Verification items for this drawing (mm, ordinates from the low corner). A direction names the side the tool comes from. Coordinates: 2 decimals unless noted, no trailing zeros. Write each loop counter-clockwise with the first axis right and the second up, starting at its lowest first coordinate (ties: lowest second). Pieces come first, ordered by that corner, then holes. Notation, with made-up numbers: M -14,66.5 L 38,66.5 A21 cw 38,81.5 Z; hole C 56,1 d7. An arc over 180 degrees is marked long. Write each question's results on one line, items separated by ' | '.
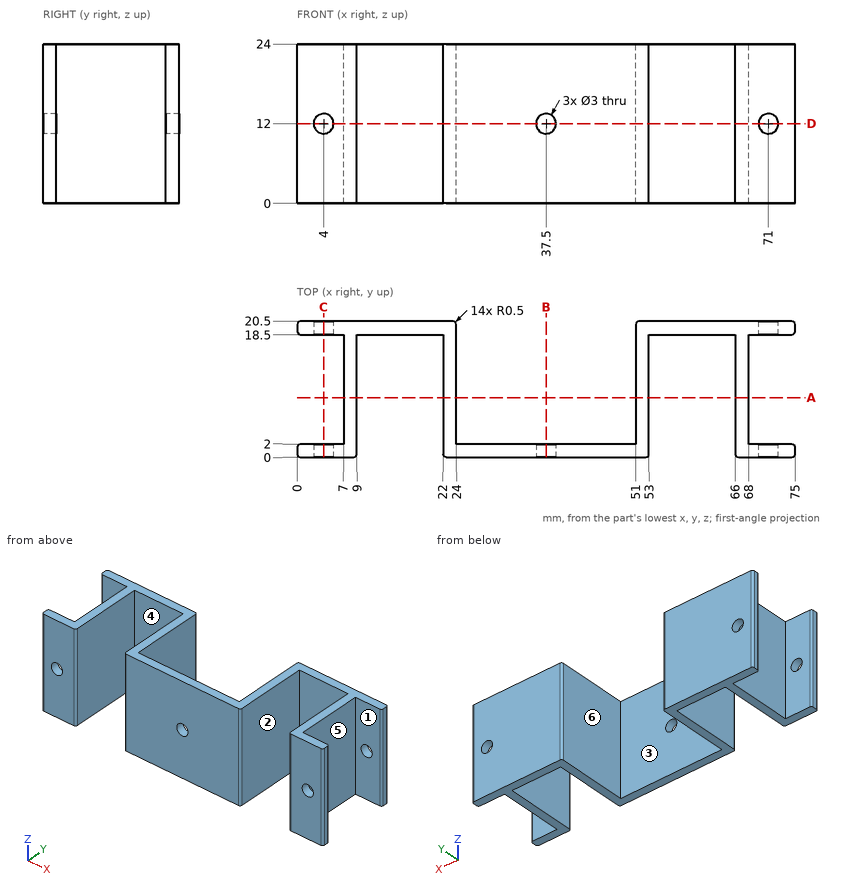
Q1. Scan lines: probe 1 along X at (y, z) = (8.5, 2); probe 2 along X at (y, z) = (1.5, 4.5); probe 3 along Z at (x, y) = (37.5, 0.85). Record each from-to range of solid material in increasing order.
Geometry check:
probe 1: x = 7 to 9, 22 to 24, 51 to 53, 66 to 68 | probe 2: x = 0 to 9, 22 to 53, 66 to 75 | probe 3: z = 0 to 10.5, 13.5 to 24
Q2. Sectioned sample at D-D on z = 12. Give the number of separate pieces and of enclosed holes in the cut face, and give its area (3 significant figures).
Geometry check:
separate pieces: 6 | enclosed holes: 0 | area: 295 mm2
Q3. Mould release check, pull along Y, two halves, no side actions. Record for the marked faces 4, 5 and 6: pulls with the +Y half, pulls with the -Y half, needs draft (parallel to the pull), parting line crosses it, or undercut.
Geometry check:
face 4: pulls with the -Y half | face 5: undercut | face 6: needs draft
Q4. Sectioned sample at A-A on y = 9. Record the cut outline in (x, z), and give its area (3 significant figures).
Geometry check:
outline: M 7,0 L 9,0 L 9,24 L 7,24 Z; M 22,0 L 24,0 L 24,24 L 22,24 Z; M 51,0 L 53,0 L 53,24 L 51,24 Z; M 66,0 L 68,0 L 68,24 L 66,24 Z | area: 192 mm2
Q5. Depth check by flat-ended pin: P1, Ø2, axis at y = 11.5, z = 15, coming from the -X side; P2, Ø8, axis at y = 8.5, z = 19.5, coming from the +X side; P3, Ø4, axis at x = 14.5, z = 7, coming from the -Y side; P4, Ø12, axis at x = 42, y = 13.5, coming from the -Z side. Enter the tip coordinate at first touch or a pass-through.
Geometry check:
P1: stops at x = 7 | P2: stops at x = 68 | P3: stops at y = 18.5 | P4: passes through
Q6. Sectioned sample at C-C on x = 4. Record the cut outline in (y, z), and give its area (3 significant figures).
Geometry check:
outline: M 0,0 L 2,0 L 2,10.5 L 0,10.5 Z; M 0,13.5 L 2,13.5 L 2,24 L 0,24 Z; M 18.5,0 L 20.5,0 L 20.5,10.5 L 18.5,10.5 Z; M 18.5,13.5 L 20.5,13.5 L 20.5,24 L 18.5,24 Z | area: 84.0 mm2
Q7. Sectioned sample at B-B on x = 37.5. Record the cut outline in (y, z), and give its area (3 significant figures).
Geometry check:
outline: M 0,0 L 2,0 L 2,10.5 L 0,10.5 Z; M 0,13.5 L 2,13.5 L 2,24 L 0,24 Z | area: 42.0 mm2
Q8. Access from +Z, -Z, +X, -X, +Y, -Y to the whole of each face (thin tool, end or side, straight path). Record for the marked faces 1, 2 and 3.
Geometry check:
face 1: +Z, -Z, +X | face 2: +Z, -Z, -Y | face 3: +Z, -Z, +Y
